Input: part model. Units: mm. Frame: model coordinates. Give positions to 0.01 mm unless a question says otherwise; leave off trailing zeros. Write each loop counter-clockwise with the first axis right and the second up, starting at its lowest first coordinate (ties: lowest second). Pieces come first, ordered by that corner, then holes. Notation, with made-up numbers: (-23.5, 28) -> (11.5, 28) arc R7 cw to (11.5, 35) -> close; hole circle Ø3 at (50.25, 9.25). An arc over 180 degrees is marked (long way). Return JSON: item names as keys, results as strings. Group by question number.
Item 1: Section A-A, the plane x = -10.5. Return loops of the section in (y, z), then the cut area to 3 significant figures.
Item 2: Line query: line 1 (Y direction, x = 3, z = -45); line 2 (Z direction, x = 18, y = 154.5). Output: solid intervals per line, ascending. Write a range as [from, to].
Item 3: Pin query (flat end, axial travel): P1, Ø22.5, axis at x = 7, y = 181.5, coming from the -Z side; P2, Ø13.5, axis at x = 9, y = 2201, coming from the +Z side. Return the tip coordinate at first contact, or that it passes through.
Solid Edge part; units mm, degrees
sketch "Sketch1" plane through (0, 0, 0) normal (0, -1, 0) x (1, 0, 0)
  line L0 (-22.5, -72.5) -> (22.5, -72.5)
  line L1 (22.5, -72.5) -> (22.5, 72.5)
  line L2 (22.5, 72.5) -> (-22.5, 72.5)
  line L3 (-22.5, 72.5) -> (-22.5, -72.5)
extrude "Protrusion1" add sketch "Sketch1" against normal blind 2370
sketch "Sketch2" plane through (22.5, 1185, 0) normal (1, 0, 0) x (0, 1, 0)
  line L0 (1035, 72.5) -> (1035, 36.25)
  line L1 (1035, 36.25) -> (990, 36.25)
  line L2 (990, 36.25) -> (990, 72.5)
  line L3 (990, 72.5) -> (1035, 72.5)
  line L4 (-1035, 72.5) -> (-1035, 36.25)
  line L5 (-1035, 36.25) -> (-990, 36.25)
  line L6 (-990, 36.25) -> (-990, 72.5)
  line L7 (-990, 72.5) -> (-1035, 72.5)
extrude "ExtrudedCutout_1" cut sketch "Sketch2" against normal blind 89.2118
mirror "Mirror1" about plane through (0, 0, 0) normal (0, 0, -1) of "ExtrudedCutout_1"
properties material "Wood, Pine"
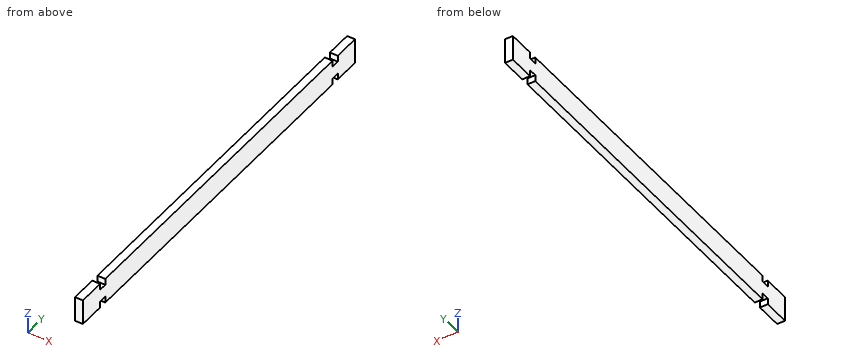
Answer below:
{
 "1": {"outline": "(0, -72.5) -> (150, -72.5) -> (150, -36.25) -> (195, -36.25) -> (195, -72.5) -> (2175, -72.5) -> (2175, -36.25) -> (2220, -36.25) -> (2220, -72.5) -> (2370, -72.5) -> (2370, 72.5) -> (2220, 72.5) -> (2220, 36.25) -> (2175, 36.25) -> (2175, 72.5) -> (195, 72.5) -> (195, 36.25) -> (150, 36.25) -> (150, 72.5) -> (0, 72.5) -> close", "area": "337,000 mm2"},
 "2": {"line 1": "y = [0, 150], [195, 2175], [2220, 2370]", "line 2": "z = [-36.25, 36.25]"},
 "3": {"P1": "stops at z = -36.25", "P2": "stops at z = 36.25"}
}
